```python
from build123d import *

# Parameters (mm, degrees)
ESQUISSE1_W        = 4.807532778
ESQUISSE1_H        = 10
ESQUISSE1_W_2      = 9.57980661
BOSS_EXTRU_1_DEPTH = 5


with BuildPart() as part:
    # Esquisse1 → Boss.-Extru.1 (new body)
    with BuildSketch(Plane.XY):
        Polygon((90, 82), (90, 167), (90, 172), (80, 172), (80, 167), (10, 167), (10, 172), (0, 172), (0, 167), (0, 0), (0, -5), (5, -5), (5, 0), (90, 0), (90, 47), (82.5, 47), (82.5, 82), align=None)
        with Locations((66.738521132, 30)):
            Rectangle(ESQUISSE1_W, ESQUISSE1_H, mode=Mode.SUBTRACT)
        with Locations((66.738521132, 10)):
            Rectangle(ESQUISSE1_W, ESQUISSE1_H, mode=Mode.SUBTRACT)
        with Locations((16.093272864, 25)):
            Rectangle(ESQUISSE1_W_2, ESQUISSE1_H, mode=Mode.SUBTRACT)
        with Locations((16.093272864, 55)):
            Rectangle(ESQUISSE1_W_2, ESQUISSE1_H, mode=Mode.SUBTRACT)
    extrude(amount=BOSS_EXTRU_1_DEPTH)


solid = part.part
```
Can you work these out from the model? Positions are in its coordinate system, mm. A direction names the side the tool comes from. Round coordinates to 2 decimals unless told otherwise and drop trailing zeros. Loops run counter-clockwise (first coordinate to the right, second up) from the corner with the lowest first, then second, coordinate; pieces in that order, holes last. Notation, with made-up numbers: (-30, -40) -> (-2, -40) arc R33 cw to (-2, -11) -> close; hole circle Ø9 at (42, 37). An arc over 180 degrees is marked (long way). One line per item, written item: value. Start each with the question number.
1. For pin 1 (1.5 mm diameter, centred on x = 15.5, z = 3, fed in from +Y); pin 2 (1.5 mm diameter, centred on x = 41.5, z = 2, fed in from -Y); pin 3 (1.5 mm diameter, centred on y = -3.5, z = 3.5, fed in from +X); pin 4 (1.5 mm diameter, centred on y = 68.5, z = 0.5, fed in from -X), each with a flat end and sliding along its axis, tell me the tip position at first contact or that it passes through.
2. If we section it at C-C, the plane y = 53.5: Write out the boundary of the cut face in (x, z), then the cut area to 3 significant figures.
3. For faces 4 (the flat face through (45, 167, 2)), 5 (the flat face through (16, 30, 2)), 6 (the flat face through (5, -3, 2)), 7 (the flat face through (86, 47, 2)), which set-ups out of +Z, -Z, +X, -X, +Y, -Y let a thin tool reach every point of the face, with its end or its side?
4. If we section it at A-A, the plane y = 32.5: Write out the boundary of the cut face in (x, z), then the cut area to 3 significant figures.
5. If I drill on probe 1 along Y at (x, z) = (67, 2.3); probe 2 along X at (y, z) = (25.5, 4.45); probe 3 along X at (y, z) = (9, 2.6), over which ranges is the centre line in solid material (lowest first)?
6. If we section it at D-D, the plane x = 73: Write out the boundary of the cut face in (y, z), then the cut area to 3 significant figures.
7. If we section it at B-B, the plane z = 3: Give the number of separate pieces and of enclosed holes in the cut face, then the cut area to 3 significant figures.
8. If we mould it in two halves opening along Y, with no side actions, what happens to faces 1 (the flat face through (5, 172, 2)), 2 (the flat face through (44, 85, 5)), 3 (the flat face through (11.303, 55, 2))? For each: pulls with the +Y half, pulls with the -Y half, needs draft (parallel to the pull), parting line crosses it, or undercut.
Calculated:
1. pin 1: stops at y = 167
1. pin 2: stops at y = 0
1. pin 3: stops at x = 5
1. pin 4: stops at x = 0
2. outline: (0, 0) -> (11.3, 0) -> (11.3, 5) -> (0, 5) -> close; (20.88, 0) -> (82.5, 0) -> (82.5, 5) -> (20.88, 5) -> close
2. area: 365 mm²
3. face 4: +Z, -Z, +Y
3. face 5: +Z, -Z
3. face 6: +Z, -Z, +X, -Y
3. face 7: +Z, -Z, +X
4. outline: (0, 0) -> (64.33, 0) -> (64.33, 5) -> (0, 5) -> close; (69.14, 0) -> (90, 0) -> (90, 5) -> (69.14, 5) -> close
4. area: 426 mm²
5. probe 1: y = 0 to 5, 15 to 25, 35 to 167
5. probe 2: x = 0 to 11.3, 20.88 to 64.33, 69.14 to 90
5. probe 3: x = 0 to 64.33, 69.14 to 90
6. outline: (0, 0) -> (167, 0) -> (167, 5) -> (0, 5) -> close
6. area: 835 mm²
7. separate pieces: 1
7. enclosed holes: 4
7. area: 14,600 mm²
8. face 1: pulls with the +Y half
8. face 2: needs draft
8. face 3: undercut
